Answer from the drawing. Dimensions are ordinates in mm from the lowest x, y and z of the part. Coordinates: 2 decimals unless noted, no trailing zeros. Order: outer loops, then holes, each group sorted by start corner. A loop starts at its lowest first (then second) coordinate and runs counter-clockwise, first axis right, second up. Notation, with made-up numbers: (71, -5.75) -> (104, -5.75) arc R20 cw to (104, 23.25) -> close; hole circle Ø5 at (-33, 25.25). An arc over 180 degrees is marked (long way). Answer in a Markdown table with one row per item.
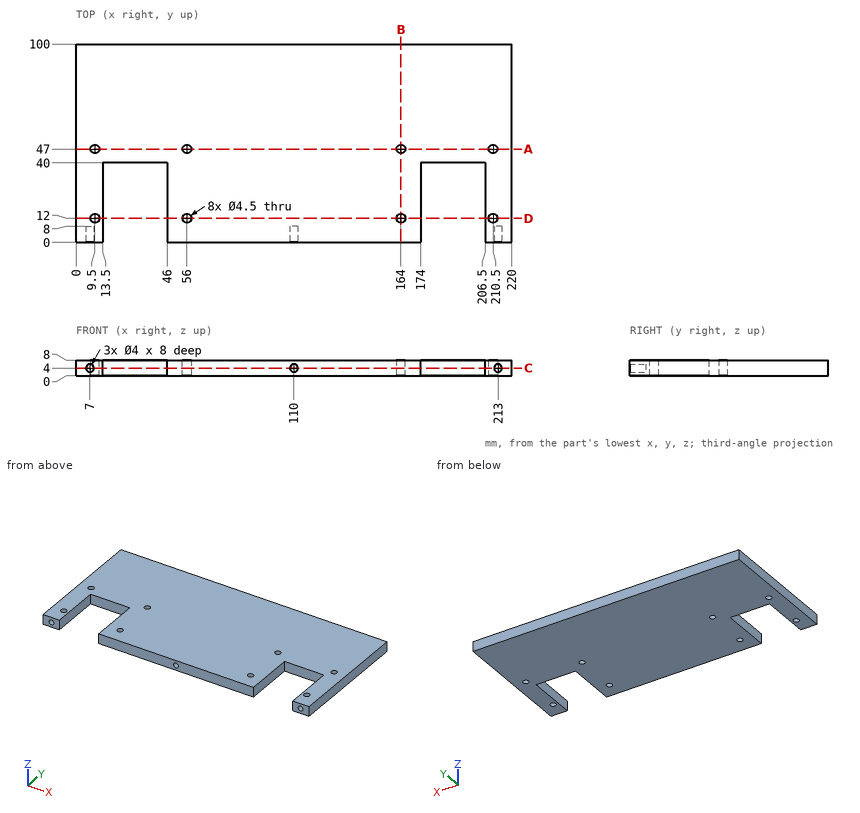
Q1. The part is cut by section C-C (z = 4). Give the number of separate pieces and of enclosed holes in the cut face, then the cut area to 3 significant figures.
Outcome:
| item | result |
|---|---|
| separate pieces | 1 |
| enclosed holes | 8 |
| area | 19,200 mm² |
Q2. The part is cut by section B-B (x = 164). Write down the section's boundary in (y, z).
Outcome:
| item | result |
|---|---|
| outline | (0, 0) -> (9.75, 0) -> (9.75, 8) -> (0, 8) -> close; (14.25, 0) -> (44.75, 0) -> (44.75, 8) -> (14.25, 8) -> close; (49.25, 0) -> (100, 0) -> (100, 8) -> (49.25, 8) -> close |
Q3. Consider line 1 (X direction, y = 4.75, z = 4); line 2 (X direction, y = 19, z = 2.5); line 3 (Y direction, x = 9.5, z = 3). Determine where each line is inside the solid, lowest interval first.
Outcome:
| item | result |
|---|---|
| line 1 | 0 to 5, 9 to 13.5, 46 to 108, 112 to 174, 206.5 to 211, 215 to 220 |
| line 2 | 0 to 13.5, 46 to 174, 206.5 to 220 |
| line 3 | 0 to 9.75, 14.25 to 44.75, 49.25 to 100 |
Q4. The part is cut by section D-D (y = 12). Write down the section's boundary in (x, z), then the cut area to 3 significant figures.
Outcome:
| item | result |
|---|---|
| outline | (0, 0) -> (7.25, 0) -> (7.25, 8) -> (0, 8) -> close; (11.75, 0) -> (13.5, 0) -> (13.5, 8) -> (11.75, 8) -> close; (46, 0) -> (53.75, 0) -> (53.75, 8) -> (46, 8) -> close; (58.25, 0) -> (161.75, 0) -> (161.75, 8) -> (58.25, 8) -> close; (166.25, 0) -> (174, 0) -> (174, 8) -> (166.25, 8) -> close; (206.5, 0) -> (208.25, 0) -> (208.25, 8) -> (206.5, 8) -> close; (212.75, 0) -> (220, 0) -> (220, 8) -> (212.75, 8) -> close |
| area | 1,100 mm² |
Q5. Given pin 1 (1.2 mm diameter, centred on x = 212, z = 4.5, fed in from -Y); pin 2 (3.5 mm diameter, centred on x = 9.5, y = 47, fed in from +Z), each flat-ended and moving along its own axis, determine where each tip first touches the part or whether it passes through.
Outcome:
| item | result |
|---|---|
| pin 1 | y = 8 |
| pin 2 | through |
Q6. The part is cut by section A-A (y = 47). Write down the section's boundary in (x, z), then the cut area to 3 significant figures.
Outcome:
| item | result |
|---|---|
| outline | (0, 0) -> (7.25, 0) -> (7.25, 8) -> (0, 8) -> close; (11.75, 0) -> (53.75, 0) -> (53.75, 8) -> (11.75, 8) -> close; (58.25, 0) -> (161.75, 0) -> (161.75, 8) -> (58.25, 8) -> close; (166.25, 0) -> (208.25, 0) -> (208.25, 8) -> (166.25, 8) -> close; (212.75, 0) -> (220, 0) -> (220, 8) -> (212.75, 8) -> close |
| area | 1,620 mm² |
